Can you work these out from the model? Positions are in its coordinate system, mm. A direction names the side the tool comes from. Round coordinates to 2 decimals unless told otherwise and drop trailing zeros. Order: outer loops, then holes, each group sorted by start corner. A loop starts at its lowest first (then second) coordinate and runs counter-clockwise, first axis right, second up. Notation, with made-up numbers: M 59,82.25 L 99,82.25 A21 cw 99,120.25 Z; hole C -16.5,-23.5 d10. An arc over 180 degrees is marked long. One line per question, with ' | ' between items.
```python
from build123d import *

# Parameters (mm, degrees)
ESQUISSE1_W                                       = 100
ESQUISSE1_H                                       = 80
BOSS_EXTRU_1_DEPTH                                = 10
ESQUISSE2_W                                       = 70
ESQUISSE2_H                                       = 80
BOSS_EXTRU_2_DEPTH                                = 28
BOSS_EXTRU_3_DEPTH                                = 6.15
ESQUISSE3_W                                       = 8
ESQUISSE3_H                                       = 4
ESQUISSE4_R                                       = 21
ENL_V_MAT_EXTRU_1_DEPTH                           = 30
ESQUISSE5_R                                       = 12.1
ENL_V_MAT_EXTRU_2_DEPTH                           = 6
ESQUISSE6_R                                       = 6.2
ENL_V_MAT_EXTRU_3_DEPTH                           = 33.0000001
ENL_V_MAT_EXTRU_5_DEPTH                           = 87.15
CHAMBRAGE_POUR_VIS_SIX_PANS_CREUX_M41_D           = 4.8
CHAMBRAGE_POUR_VIS_SIX_PANS_CREUX_M41_CBORE_D     = 8
CHAMBRAGE_POUR_VIS_SIX_PANS_CREUX_M41_CBORE_DEPTH = 4.4
CONG_1_R                                          = 2


with BuildPart() as part:
    # Esquisse1 → Boss.-Extru.1 (new body)
    with BuildSketch(Plane(origin=(0, 0, 0), x_dir=(1, 0, 0), z_dir=(0, 1, 0))):
        with Locations((50, 40)):
            Rectangle(ESQUISSE1_W, ESQUISSE1_H)
    extrude(amount=BOSS_EXTRU_1_DEPTH)

    # Esquisse2 → Boss.-Extru.2 (add)
    with BuildSketch(Plane.XZ):
        with Locations((50, -40)):
            Rectangle(ESQUISSE2_W, ESQUISSE2_H)
    extrude(amount=BOSS_EXTRU_2_DEPTH)

    # Esquisse11 → Boss.-Extru.3 (add)
    with BuildSketch(Plane(origin=(0, 0, -80), x_dir=(-1, 0, 0), z_dir=(0, 0, -1))):
        with BuildLine():
            Line((-70, -28), (-30, -28))
            ThreePointArc((-30, -28), (-50, -8), (-70, -28))
        make_face()
    extrude(amount=BOSS_EXTRU_3_DEPTH)

    # Esquisse3 → Enlèvement de matière-Révolution1 (revolve, cut)
    with BuildSketch(Plane(origin=(0, -28, -30), x_dir=(1, 0, 0), z_dir=(0, 1, 0))):
        with Locations((54, -28)):
            Rectangle(ESQUISSE3_W, ESQUISSE3_H)
        Polygon((58, -19.8), (50, -19.8), (50, -26), (58, -26), (62, -26), (62, -19.8), align=None)
        with Locations((54, -17.8)):
            Rectangle(ESQUISSE3_W, ESQUISSE3_H)
        Polygon((58, 41.95), (50, 41.95), (50, -15.8), (58, -15.8), (71.5, -15.8), (71.5, 41.95), align=None)
        with Locations((54, 43.95)):
            Rectangle(ESQUISSE3_W, ESQUISSE3_H)
        Polygon((62, 52.15), (50, 52.15), (50, 45.95), (58, 45.95), (62, 45.95), align=None)
    revolve(axis=Axis((50, -28, -86.15), (0, 0, 1)), mode=Mode.SUBTRACT)

    # Esquisse4 → Enlèv. mat.-Extru.1 (cut)
    with BuildSketch(Plane(origin=(0, -28, 0), x_dir=(-1, 0, 0), z_dir=(0, -1, 0))):
        with Locations((-50, 50)):
            Circle(ESQUISSE4_R)
    extrude(amount=-ENL_V_MAT_EXTRU_1_DEPTH, mode=Mode.SUBTRACT)

    # Esquisse5 → Enlèv. mat.-Extru.2 (cut)
    with BuildSketch(Plane(origin=(0, 10, 0), x_dir=(1, 0, 0), z_dir=(0, 1, 0))):
        with Locations((50, 50)):
            Circle(ESQUISSE5_R)
    extrude(amount=-ENL_V_MAT_EXTRU_2_DEPTH, mode=Mode.SUBTRACT)

    # Esquisse6 → Enlèv. mat.-Extru.3 (cut, through all)
    with BuildSketch(Plane(origin=(0, 4, 0), x_dir=(1, 0, 0), z_dir=(0, 1, 0))):
        with Locations((50, 50)):
            Circle(ESQUISSE6_R)
    extrude(amount=-ENL_V_MAT_EXTRU_3_DEPTH, mode=Mode.SUBTRACT)

    # Esquisse7 → Enlèv. mat.-Extru.5 (cut, through all)
    with BuildSketch(Plane.XY):
        with BuildLine():
            Line((24.656854249, -19.656854249), (18.292893219, -13.292893219))
            ThreePointArc((18.292893219, -13.292893219), (17.96846987, -13.076120467), (17.585786438, -13))
            Line((17.585786438, -13), (15, -13))
            Line((15, -13), (15, -28))
            Line((15, -28), (18, -28))
            Line((18, -28), (18, -19.656854249))
            ThreePointArc((18, -19.656854249), (18.617316568, -18.732974717), (19.707106781, -18.949747468))
            Line((19.707106781, -18.949747468), (22.535533906, -21.778174593))
            ThreePointArc((22.535533906, -21.778174593), (23.242640687, -22.071067812), (23.949747468, -21.778174593))
            Line((23.949747468, -21.778174593), (24.656854249, -21.071067812))
            ThreePointArc((24.656854249, -21.071067812), (24.949747468, -20.363961031), (24.656854249, -19.656854249))
        make_face()
        with BuildLine():
            Line((82, -19.656854249), (82, -28))
            Line((82, -28), (85, -28))
            Line((85, -28), (85, -13))
            Line((85, -13), (82.414213562, -13))
            ThreePointArc((82.414213562, -13), (82.03153013, -13.076120467), (81.707106781, -13.292893219))
            Line((81.707106781, -13.292893219), (75.343145751, -19.656854249))
            ThreePointArc((75.343145751, -19.656854249), (75.050252532, -20.363961031), (75.343145751, -21.071067812))
            Line((75.343145751, -21.071067812), (76.050252532, -21.778174593))
            ThreePointArc((76.050252532, -21.778174593), (76.757359313, -22.071067812), (77.464466094, -21.778174593))
            Line((77.464466094, -21.778174593), (80.292893219, -18.949747468))
            ThreePointArc((80.292893219, -18.949747468), (81.382683432, -18.732974717), (82, -19.656854249))
        make_face()
    extrude(amount=-ENL_V_MAT_EXTRU_5_DEPTH, mode=Mode.SUBTRACT)

    # Chambrage pour vis à six pans creux M41 (through all)
    with Locations(Plane(origin=(7.5, 0, -10), x_dir=(0, 0, -1), z_dir=(0, -1, 0))):
        with Locations((0, 0), (60, 0), (60, 85), (0, 85)):
            CounterBoreHole(CHAMBRAGE_POUR_VIS_SIX_PANS_CREUX_M41_D / 2, CHAMBRAGE_POUR_VIS_SIX_PANS_CREUX_M41_CBORE_D / 2, CHAMBRAGE_POUR_VIS_SIX_PANS_CREUX_M41_CBORE_DEPTH)

    # Congé1
    cong_1_edges = [part.edges().sort_by_distance(p)[0] for p in [
        (92.5, 0, 0),
        (92.5, 0, -80),
        (15, 0, -40),
        (85, 0, -40),
        (50, -8, -80),
        (50, -8, -86.15),
        (0, 0, -40),
        (7.5, 0, -80),
        (100, 0, -40),
        (7.5, 0, 0),
        (0, 5, 0),
        (0, 5, -80),
        (100, 5, -80),
        (100, 5, 0),
        (85, -6.5, 0),
        (85, -6.5, -80),
        (15, -6.5, -80),
        (15, -6.5, 0),
    ]]
    fillet(cong_1_edges, radius=CONG_1_R)


solid = part.part
```
(1) Please list where these lines run through material, in increasing order: probe 1 along X at (y, z) = (8, -70); probe 2 along X at (y, z) = (1.95, -10); probe 3 along X at (y, z) = (-10, -50). Write a range as [from, to].
Final values:
probe 1: [0, 5.1], [9.9, 90.1], [94.9, 100] | probe 2: [0, 3.5], [11.5, 88.5], [96.5, 100] | probe 3: [15, 29], [71, 85]
(2) On a 3-axis mill with a long thin cutter (end or side, diameter ignored), from which of +Z, -Z, +X, -X, +Y, -Y can I reach the whole of each face in a straight line? I mean faces 1 (the flat face through (50, -19, -75.95)), 2 (the cylindrical face through (6.581, 7.239, -67.783)), 3 (the flat face through (47, 4, -56)), 4 (the flat face through (15, -7, -41)), 5 (the cylindrical face through (50, -8, -83)). Say none if no direction works.
Final values:
face 1: -Y | face 2: +Y, -Y | face 3: +Y | face 4: +Z, -Z, -X, -Y | face 5: -Z, +Y
(3) If we section it at C-C on y = -4: Please give me the cut outline in (x, z).
Final values:
outline: M 15,-78 A2 ccw 17,-80 L 83,-80 A2 ccw 85,-78 L 85,-2 A2 ccw 83,0 L 17,0 A2 ccw 15,-2 Z; hole C 50,-50 d42
(4) Thinking about a two-plate mould opening in Z: for faces 6 (the flat face through (49, -5, -80)), 7 (the cylindrical face through (56.505, 7.042, -60.203)), 8 (the cylindrical face through (50, -20, -2)), which applies, released by +Z, released by -Z, zero draft, split by the parting line, or undercut?
Final values:
face 6: released by -Z | face 7: undercut | face 8: zero draft
(5) If we section it at B-B on x = 7.5: Please give me the cut outline in (y, z), plus the area to 3 significant figures.
Final values:
outline: M 0,-78 A2 ccw 2,-80 L 10,-80 L 10,-72.4 L 4.4,-72.4 L 4.4,-74 L 0,-74 Z; M 0,-66 L 4.4,-66 L 4.4,-67.6 L 10,-67.6 L 10,-12.4 L 4.4,-12.4 L 4.4,-14 L 0,-14 Z; M 0,-6 L 4.4,-6 L 4.4,-7.6 L 10,-7.6 L 10,0 L 2,0 A2 ccw 0,-2 Z | area: 674 mm^2
(6) Will these pins go through, and if not, where does the flat tip stop? pin 1 Ø5 at (x, y) = (31, -18) entering from -Z; pin 2 Ø1 at (x, z) = (90, -26.5) entering from -Y; pin 3 Ø1.3 at (x, z) = (16, -45.5) entering from -Y; pin 4 Ø2.5 at (x, z) = (91.5, -70) entering from -Y.
Final values:
pin 1: z = -85.9 | pin 2: y = 0 | pin 3: y = -13 | pin 4: through
